Build history of the part. All positions in model axes, mm. Face numbers are marked on the shaded views. Coordinates: 2 decimals unless noted, no trailing zeros. Loops run counter-clockwise (first coordinate to the right, second up) from the corner with the lowest first, then second, coordinate; pieces in that order, holes last. Notation, with made-up numbers: (36, 27) -> (74, 27) arc R32 ccw to (74, 54) -> close; hole circle Ø10 at (10, 89). An arc over 180 degrees is marked (long way). One line per item, written item: value. Start each with the question number.
```python
from build123d import *

# Parameters (mm, degrees)
BOSS_EXTRUDE1_DEPTH     = 4.8
SKETCH2_R               = 1.55
CUT_EXTRUDE1_DEPTH      = 4.8
MIRROR2_COPY_1_SKETCH_R = 1.55
MIRROR2_COPY_1_DEPTH    = 4.8
FILLET1_R               = 10


with BuildPart() as part:
    # Sketch1 → Boss-Extrude1 (new body)
    with BuildSketch(Plane(origin=(0, 0, 0), x_dir=(1, 0, 0), z_dir=(0, 1, 0))):
        Polygon((60, 150), (-60, 150), (-60, 45), (-85, 45), (-85, -45), (-60, -45), (-60, -150), (60, -150), (60, -45), (85, -45), (85, 45), (60, 45), align=None)
    extrude(amount=BOSS_EXTRUDE1_DEPTH)

    # Sketch2 → Cut-Extrude1 (cut)
    with BuildSketch(Plane(origin=(0, 4.8, 0), x_dir=(1, 0, 0), z_dir=(0, 1, 0))):
        with Locations(Location((56.003512962, -76.642970185, 0), (0, 0, 270))):
            Circle(SKETCH2_R)
        with Locations(Location((49.903512962, -76.642970185, 0), (0, 0, 270))):
            Circle(SKETCH2_R)
        with Locations(Location((56.003512962, -106.542970185, 0), (0, 0, 270))):
            Circle(SKETCH2_R)
        with Locations(Location((49.903512962, -106.542970185, 0), (0, 0, 270))):
            Circle(SKETCH2_R)
        with Locations(Location((43.803512962, -76.642970185, 0), (0, 0, 270))):
            Circle(SKETCH2_R)
        with Locations(Location((43.803512962, -106.542970185, 0), (0, 0, 270))):
            Circle(SKETCH2_R)
    cut_extrude1 = extrude(amount=-CUT_EXTRUDE1_DEPTH, mode=Mode.SUBTRACT)

    # Mirror1: Cut-Extrude1 across plane
    add(cut_extrude1.mirror(Plane(origin=(0, 0, 0), x_dir=(0, 0, 1), z_dir=(1, 0, 0))), mode=Mode.SUBTRACT)

    # Mirror2: Cut-Extrude1 across plane
    add(cut_extrude1.mirror(Plane.XY), mode=Mode.SUBTRACT)

    # Mirror2 copy 1 sketch → Mirror2 copy 1 (cut)
    with BuildSketch(Plane(origin=(0, 4.8, 0), x_dir=(-1, 0, 0), z_dir=(0, 1, 0))):
        with Locations(Location((56.003512962, -76.642970185, 0), (0, 0, 270))):
            Circle(MIRROR2_COPY_1_SKETCH_R)
        with Locations(Location((49.903512962, -76.642970185, 0), (0, 0, 270))):
            Circle(MIRROR2_COPY_1_SKETCH_R)
        with Locations(Location((56.003512962, -106.542970185, 0), (0, 0, 270))):
            Circle(MIRROR2_COPY_1_SKETCH_R)
        with Locations(Location((49.903512962, -106.542970185, 0), (0, 0, 270))):
            Circle(MIRROR2_COPY_1_SKETCH_R)
        with Locations(Location((43.803512962, -76.642970185, 0), (0, 0, 270))):
            Circle(MIRROR2_COPY_1_SKETCH_R)
        with Locations(Location((43.803512962, -106.542970185, 0), (0, 0, 270))):
            Circle(MIRROR2_COPY_1_SKETCH_R)
    extrude(amount=-MIRROR2_COPY_1_DEPTH, mode=Mode.SUBTRACT)

    # Fillet1
    fillet1_edges = [part.edges().sort_by_distance(p)[0] for p in [
        (85, 2.4, -45),
        (85, 2.4, 45),
        (60, 2.4, 150),
        (-60, 2.4, 150),
        (-85, 2.4, 45),
        (-85, 2.4, -45),
        (-60, 2.4, -150),
        (60, 2.4, -150),
    ]]
    fillet(fillet1_edges, radius=FILLET1_R)


solid = part.part
```
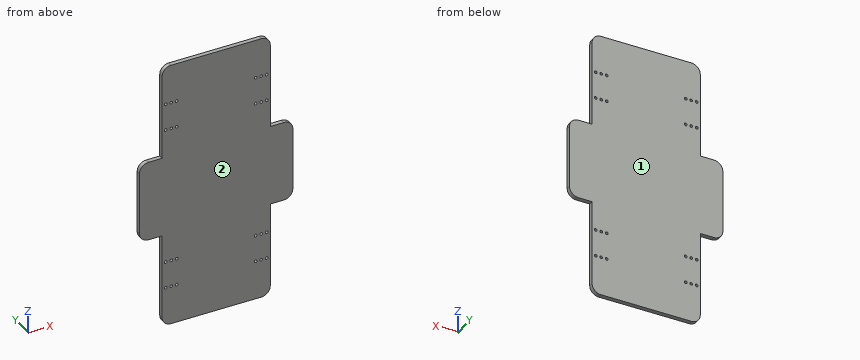
Item 1: Band-saw the part on A-A, the plane z = -88.5. List the corners of the cut face in (x, y).
Item 2: Band-saw the part on C-C, the plane y = 3.95. Count the separate pieces of the cut face and the enclosed holes in it, and give its area (3 significant figures).
Item 3: Band-saw the part on B-B, the plane x = 71. List the corners of the cut face in (y, z).
Item 4: Probe probe 1 along X at (y, z) = (4.2, -82); probe 2 along Z at (x, y) = (-73, 1.1); probe 3 along Z at (x, y) = (59, 2.8). List the from-to ranges inside material, lowest first.
Item 5: Drop flat-ended pins along their axis: pin 1 Ø2.5 at (x, y) = (-65, 3.5) entering from +Z; pin 2 Ø1.9 at (x, z) = (-49.9, 76.64) entering from +Y; pin 3 Ø1.4 at (x, y) = (66.5, 2) entering from -Z; pin 4 Ø3.5 at (x, z) = (-49.9, -76.64) entering from +Y. Give the stop position or say it passes through.
Item 6: Two-plate mould, pull along Y, no slides. Class the marked faces 1 and 2: +Y half, -Y half, draft (parallel to the pull), parting line (faces both ways), or undercut.
Worked out:
1. outline: (-60, 0) -> (60, 0) -> (60, 4.8) -> (-60, 4.8) -> close
2. separate pieces: 1
2. enclosed holes: 24
2. area: 40,100 mm²
3. outline: (0, -45) -> (4.8, -45) -> (4.8, 45) -> (0, 45) -> close
4. probe 1: x = -60 to 60
4. probe 2: z = -45 to 45
4. probe 3: z = -144.36 to 144.36
5. pin 1: stops at z = 45
5. pin 2: passes through
5. pin 3: stops at z = -45
5. pin 4: stops at y = 4.8
6. face 1: +Y half
6. face 2: -Y half
